Can you work these out from the drawing? Everything is in mm from the part's minimum corner. Give positions to 0.01 mm unless a question says otherwise; leave off trailing zeros. Loops run counter-clockwise (first coordinate to the right, second up) from the corner with the lowest first, then second, coordinate; pieces in that order, holes last. Notation, with made-up numbers: (46, 83.5) - (77, 83.5) arc R32 cw to (77, 117.5) - close; hole circle Ø3 at (-35.75, 42.5). An arc over 180 degrees is marked (long way). Answer in a Markdown table with one row per item. Add a question column.
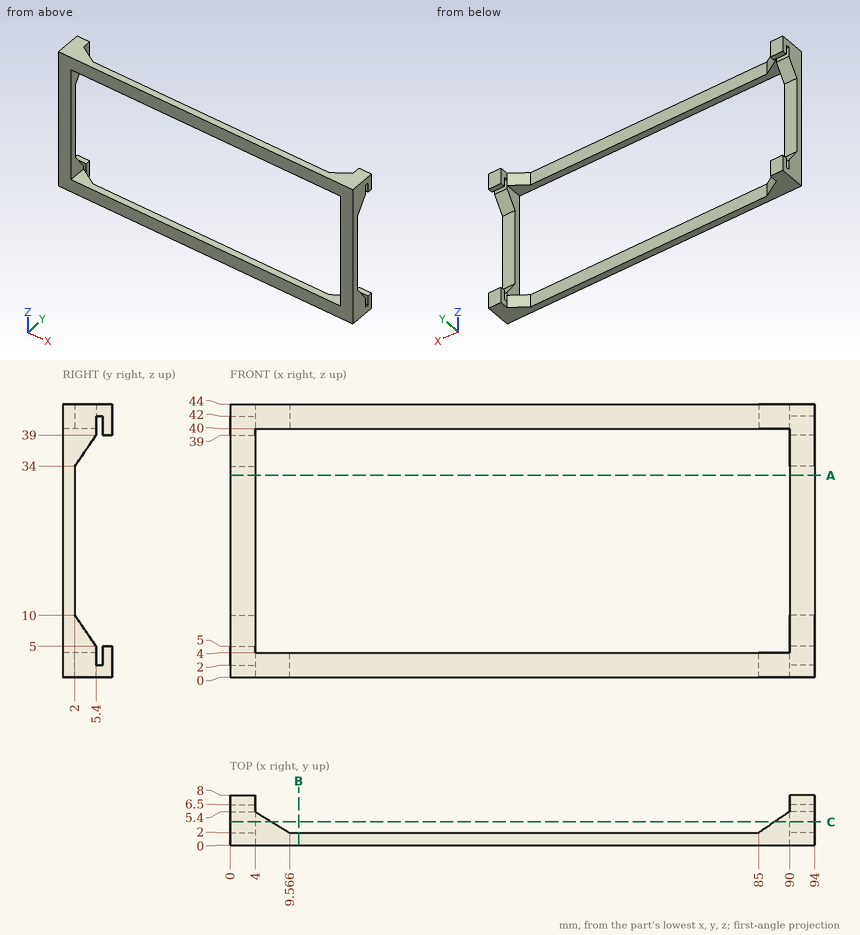
(1) I want a section at C-C on y = 3.75. Please give me the cut outline in (x, z).
(2) Please list where these lines run through material, in increasing order: line 1 (X direction, y = 0.5, z = 24); line 2 (Z direction, x = 35, y = 0.5).
(3) I want a section at B-B on x = 11. Please give me the cut outline in (y, z), then the cut area to 3 significant figures.
(4) For pin 1 Ø4 at (y, z) = (6, 36) entering from -X; pin 2 Ø3 at (x, z) = (33.5, 2.5) entering from +Y, each with a flat end and sliding along its axis, tell me the tip position at first contact or that it passes through.
(5) I want a section at A-A on z = 32.5. Please give me the cut outline in (x, y).
Reported:
| question | item | result |
|---|---|---|
| 1 | outline | (0, 0) - (6.7, 0) - (6.7, 4) - (4, 4) - (4, 7.43) - (0, 7.43) - close; (0, 36.57) - (4, 36.57) - (4, 40) - (6.7, 40) - (6.7, 44) - (0, 44) - close; (87.57, 0) - (94, 0) - (94, 7.43) - (90, 7.43) - (90, 4) - (87.57, 4) - close; (87.57, 40) - (90, 40) - (90, 36.57) - (94, 36.57) - (94, 44) - (87.57, 44) - close |
| 2 | line 1 | 0 to 4, 90 to 94 |
| 2 | line 2 | 0 to 4, 40 to 44 |
| 3 | outline | (0, 0) - (2, 0) - (2, 4) - (0, 4) - close; (0, 40) - (2, 40) - (2, 44) - (0, 44) - close |
| 3 | area | 16.0 mm² |
| 4 | pin 1 | through |
| 4 | pin 2 | y = 2 |
| 5 | outline | (0, 0) - (4, 0) - (4, 2) - (0, 2) - close; (90, 0) - (94, 0) - (94, 2) - (90, 2) - close |
